Verification items for the finished model (mm, model axes). A direction names the side the tool comes from. Round coordinates to 2 decimals unless told otherwise and drop trailing zeros. Loops run counter-clockwise (first coordinate to the right, second up) from the corner with the lowest first, then second, coordinate; pieces in that order, holes last. Notation, with made-up numbers: (61.25, 48.5) - (74.25, 48.5) arc R31 ccw to (74.25, 76.5) - close; hole circle Ø11 at (66.25, 29.25). An arc over 180 degrees is marked (long way). Use CSV: the item, a comma, the result in double quotes.
```python
from build123d import *

# Parameters (mm, degrees)
BOSS_EXTRUDE1_DEPTH = 5
FILLET1_R           = 1


with BuildPart() as part:
    # Sketch1 → Boss-Extrude1 (new body)
    with BuildSketch(Plane.XY):
        Polygon((0, 2.5), (15, 2.5), (15, -1.5), (14, -1.5), (12.75, 0), (0, 0), align=None)
    extrude(amount=BOSS_EXTRUDE1_DEPTH)

    # Fillet1
    # the kernel refuses this fillet: 1 mm, written as the material it adds along each edge
    with BuildSketch(Plane(origin=(12.75, 0, 0), x_dir=(0.6401843996644788, -0.7682212795973767, 0), z_dir=(0, 0, 1))) as fillet1_piece_1:
        with BuildLine():
            CenterArc((FILLET1_R * 0.468374945984, -FILLET1_R), FILLET1_R, 90, 50.194428908)
            Line((-FILLET1_R * 0.299846333613, -FILLET1_R * 0.359815600336), (0, 0))
            Line((0, 0), (FILLET1_R * 0.468374945984, 0))
        make_face()
    extrude(amount=5)
    # the kernel refuses this fillet: 1 mm, written as the material it takes off along each edge
    with BuildSketch(Plane(origin=(15, 2.5, -2.5), x_dir=(-1, 0, 0), z_dir=(0, 0, 1)), Plane(origin=(15, -1.5, -2.5), x_dir=(0, 1, 0), z_dir=(0, 0, 1))) as fillet1_2_piece_1:
        with BuildLine():
            CenterArc((FILLET1_R, FILLET1_R), FILLET1_R, 180, 90)
            Line((0, FILLET1_R), (0, 0))
            Line((0, 0), (FILLET1_R, 0))
        make_face()
    extrude(amount=10, mode=Mode.SUBTRACT)
    with BuildSketch(Plane(origin=(14, -1.5, -1.170937365), x_dir=(1, 0, 0), z_dir=(0, 0, 1))) as fillet1_2_piece_2:
        with BuildLine():
            CenterArc((FILLET1_R * 0.468374945984, FILLET1_R), FILLET1_R, 219.805571092, 50.194428908)
            Line((-FILLET1_R * 0.299846333613, FILLET1_R * 0.359815600336), (0, 0))
            Line((0, 0), (FILLET1_R * 0.468374945984, 0))
        make_face()
    extrude(amount=7.34187473, mode=Mode.SUBTRACT)


solid = part.part
```
1) Cross-section at A-A, the plane z = 0.6. Record the cut outline in (x, y).
Returned:
outline,"(0, 0) - (12.28, 0) arc R1 cw to (13.05, -0.36) - (13.7, -1.14) arc R1 ccw to (14.23, -1.47) arc R1 ccw to (15, -0.5) - (15, 1.5) arc R1 ccw to (14, 2.5) - (0, 2.5) - close"
2) Access from +Z, -Z, +X, -X, +Y, -Y to the whole of each face (thin tool, end or side, straight path). Record for faces 1 (the face through (14.8, -1.1, 2.5)), 2 (the face through (6, 0, 2)).
Returned:
face 1,"+Z, -Z, +X, -Y"
face 2,"+Z, -Z, -X, -Y"
3) Gauge pin test, flat end, axial feed: pin 1 Ø1 at (y, z) = (0.5, 3) entering from -X. Record the tip position at first contact, or that the pin passes through.
Returned:
pin 1,"stops at x = 0"
4) Thickness scan on probe 1 along Y at (x, z) = (1.75, 3.2); probe 2 along Y at (x, z) = (14.75, 1.05); probe 3 along X at (y, z) = (2.05, 3.7). Record the ranges inside material, lowest first. Write a range as [from, to].
Returned:
probe 1,"y = [0, 2.5]"
probe 2,"y = [-1.16, 2.16]"
probe 3,"x = [0, 14.84]"
5) Cross-section at C-C, the plane y = -0.95. Record the cut outline in (x, z).
Returned:
outline,"(13.54, 0) - (14.89, 0) - (14.89, 5) - (13.54, 5) - close"
6) Cross-section at B-B, the plane x = 10.75. Record the cut outline in (y, z).
Returned:
outline,"(0, 0) - (2.5, 0) - (2.5, 5) - (0, 5) - close"
